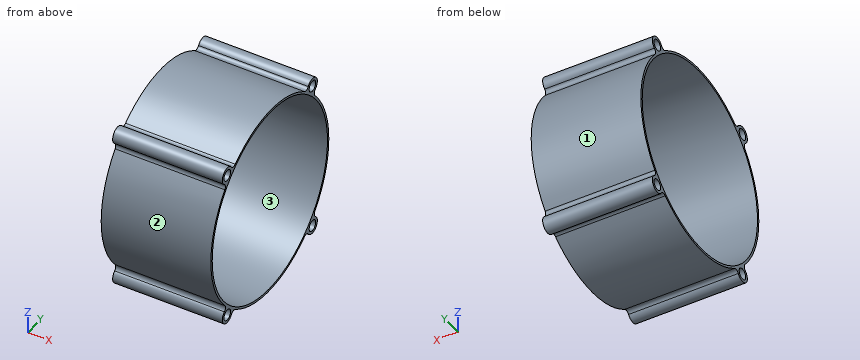
from build123d import *

# Parameters (mm, degrees)
SKETCH1_R           = 45
SKETCH1_R_2         = 44
SKETCH1_R_3         = 3.762432936
SKETCH1_R_4         = 2.5
BOSS_EXTRUDE5_DEPTH = 50
SKETCH2_R           = 2.5
CUT_EXTRUDE1_DEPTH  = 50
FILLET1_R           = 2


with BuildPart() as part:
    # Sketch1 → Boss-Extrude5 (new body)
    # profile 1 of 5: a face of its own
    with BuildSketch(Plane(origin=(0, 0, 0), x_dir=(0, 0, -1), z_dir=(1, 0, 0))):
        Circle(SKETCH1_R)
        Circle(SKETCH1_R_2, mode=Mode.SUBTRACT)
    # profile 2 of 5: a face of its own
    with BuildSketch(Plane(origin=(0, 0, 0), x_dir=(0, 0, -1), z_dir=(1, 0, 0))):
        with Locations((-35, 32.5)):
            Circle(SKETCH1_R_3)
        with Locations((-35, 32.5)):
            Circle(SKETCH1_R_4, mode=Mode.SUBTRACT)
    # profile 3 of 5: a face of its own
    with BuildSketch(Plane(origin=(0, 0, 0), x_dir=(0, 0, -1), z_dir=(1, 0, 0))):
        with Locations((-35, -32.5)):
            Circle(SKETCH1_R_3)
        with Locations((-35, -32.5)):
            Circle(SKETCH1_R_4, mode=Mode.SUBTRACT)
    # profile 4 of 5: a face of its own
    with BuildSketch(Plane(origin=(0, 0, 0), x_dir=(0, 0, -1), z_dir=(1, 0, 0))):
        with Locations((35, -32.5)):
            Circle(SKETCH1_R_3)
    # profile 5 of 5: a face of its own
    with BuildSketch(Plane(origin=(0, 0, 0), x_dir=(0, 0, -1), z_dir=(1, 0, 0))):
        with Locations((35, 32.5)):
            Circle(SKETCH1_R_3)
        with Locations((35, 32.5)):
            Circle(SKETCH1_R_4, mode=Mode.SUBTRACT)
    extrude(amount=BOSS_EXTRUDE5_DEPTH)

    # Sketch2 → Cut-Extrude1 (cut)
    with BuildSketch(Plane(origin=(50, 0, 0), x_dir=(0, 0, -1), z_dir=(1, 0, 0))):
        with Locations((35, -32.5)):
            Circle(SKETCH2_R)
    extrude(amount=-CUT_EXTRUDE1_DEPTH, mode=Mode.SUBTRACT)

    # Fillet1
    fillet1_edges = [part.edges().sort_by_distance(p)[0] for p in [
        (25, -28.757613043, 34.612132151),
        (25, 28.757613043, 34.612132151),
        (25, 32.390028906, 31.239174564),
        (25, -32.390028906, 31.239174564),
        (25, 28.757613043, -34.612132151),
        (25, 32.390028906, -31.239174564),
        (25, -32.390028906, -31.239174564),
        (25, -28.757613043, -34.612132151),
    ]]
    fillet(fillet1_edges, radius=FILLET1_R)


solid = part.part
Geometry: final body of the model. Coordinates: model frame, mm. Face numbers are marked on the shaded views. Give positions to 0.01 mm unless a question says otherwise; leave off trailing zeros. Write each loop counter-clockwise with the first axis right and the second up, starting at its lowest first coordinate (ties: lowest second). Pieces come first, ordered by that corner, then holes.
(1) Cut plane A-A, the plane z = 0. Return loops of the section in (x, y), then the cut area to 4 significant figures.
(2) Cut plane D-D, the plane y = 32.5. Return loops of the section in (x, z).
(3) First-contact query: P1, Ø4, axis at x = 33.5, z = 5, coming from the -Y side; P2, Ø1, axis at x = 36.5, y = 34, coming from the +Z side; P3, Ø10, axis at x = 15.5, z = 21, coming from the +Y side. Flat tips, straight axial feed; report the tip coordinate or a pass-through.
(4) Cut plane C-C, the plane x = 19. Give the number of separate pieces and of enclosed holes in the cut face, then the cut area to 3 significant figures.
(5) Mould query, pull axis Y, two halves, no side actions, for the marked faces 1, 2 and 3. Classes: released by +Y, released by -Y, zero draft, split by the parting line, or undercut.
(6) Cut plane B-B, the plane y = -15.5. Return loops of the section in (x, z), then the cut area to 3 significant figures.
(7) Ray query, line 1 (Y direction, x = 40, z = 0); line 2 (Y direction, x = 33, z = -35); line 3 (Z direction, x = 7, y = -8). Return the intervals inside material, ascending.
Values follow:
1. outline: (0, -45) - (50, -45) - (50, -44) - (0, -44) - close; (0, 44) - (50, 44) - (50, 45) - (0, 45) - close
1. area: 100.0 mm2
2. outline: (0, -38.76) - (50, -38.76) - (50, -37.5) - (0, -37.5) - close; (0, -32.5) - (50, -32.5) - (50, -29.66) - (0, -29.66) - close; (0, 29.66) - (50, 29.66) - (50, 32.5) - (0, 32.5) - close; (0, 37.5) - (50, 37.5) - (50, 38.76) - (0, 38.76) - close
3. P1: stops at y = -44.9
3. P2: stops at z = 38.63
3. P3: stops at y = 42.06
4. separate pieces: 1
4. enclosed holes: 5
4. area: 378 mm2
5. face 1: released by +Y
5. face 2: released by -Y
5. face 3: undercut
6. outline: (0, -42.25) - (50, -42.25) - (50, -41.18) - (0, -41.18) - close; (0, 41.18) - (50, 41.18) - (50, 42.25) - (0, 42.25) - close
6. area: 107 mm2
7. line 1: y = -45 to -44, 44 to 45
7. line 2: y = -36.26 to -35, -30 to -26.66, 26.66 to 30, 35 to 36.26
7. line 3: z = -44.28 to -43.27, 43.27 to 44.28
